Part print with two shaded views. Sizes in mm from the minimum x, y, z corner. A direction names the side the tool comes from. Round coordinates to 2 decimals unless told otherwise and drop trailing zeros. Order: outer loops, then holes, each group sorted by start corner. A loop starts at its lowest first (then second) coordinate and runs counter-clockwise, first axis right, second up. Notation, with made-up numbers: (79, -39) - (113, -39) arc R6 ccw to (113, -32) - close; hole circle Ø9 at (16, 18.5). An arc over 180 degrees is marked (long way). Use one line per item in the form item = value.
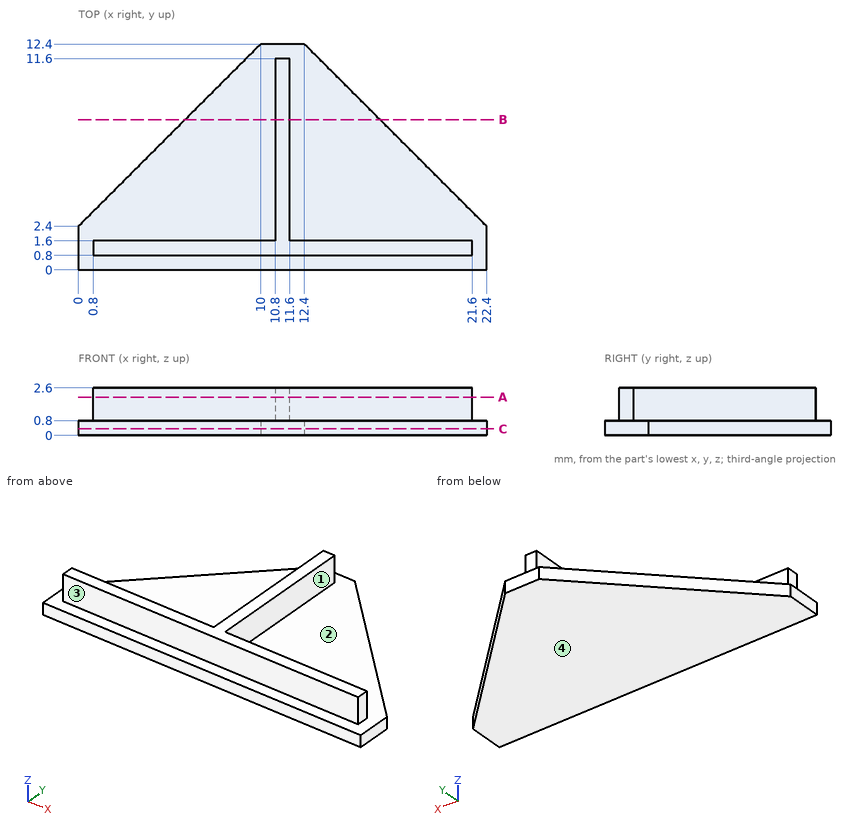
(1) Slice it at A-A on z = 2.1. Give the cut face in (x, y).
Report:
outline = (0.8, 0.8) - (21.6, 0.8) - (21.6, 1.6) - (11.6, 1.6) - (11.6, 11.6) - (10.8, 11.6) - (10.8, 1.6) - (0.8, 1.6) - close
(2) Probe probe 1 along X at (y, z) = (6.25, 1.55); probe 2 along Y at (x, z) = (10.5, 2.55); probe 3 along Z at (x, y) = (21.5, 2.75). List the from-to ranges inside material, lowest first. Write a range as [from, to].
Report:
probe_1 = [10.8, 11.6]
probe_2 = [0.8, 1.6]
probe_3 = [0, 0.8]
(3) Slice it at B-B on y = 8.25. Give the cut face in (x, z).
Report:
outline = (5.85, 0) - (16.55, 0) - (16.55, 0.8) - (11.6, 0.8) - (11.6, 2.6) - (10.8, 2.6) - (10.8, 0.8) - (5.85, 0.8) - close
(4) Pin check, flat tips, straight feed: pin 1 (3.5 mm diameter, centred on x = 7, y = 8.5, fed in from +Z); pin 2 (0.6 mm diameter, centred on y = 1, z = 1.5, fed in from +X); pin 3 (0.9 mm diameter, centred on y = 1, z = 2, fed in from -X). Stop position of each tip, or through.
Report:
pin_1 = 0.8
pin_2 = 21.6
pin_3 = 0.8
(5) Slice it at C-C on z = 0.35. Give the cut face in (x, y).
Report:
outline = (0, 0) - (22.4, 0) - (22.4, 2.4) - (12.4, 12.4) - (10, 12.4) - (0, 2.4) - close
(6) Tool access for the marked faces 1, 2, 3 and 4: list every direction of +Z, -Z, +X, -X, +Y, -Y with a clear straight run to the whole face (end or side of a thin tool).
Report:
face_1 = +Z, +X, +Y
face_2 = +Z
face_3 = +Z, +X, -X, -Y
face_4 = -Z, +X, -X, +Y, -Y
